Design review of the part shown in the three views and the two pictorial views. Dimensions are in mm from the part's minimum x, y and z. A direction names the side the tool comes from. Coordinates: 2 decimals unless noted, no trailing zeros. Loops run counter-clockwise (first coordinate to the right, second up) from the corner with the lowest first, then second, coordinate; pieces in that order, holes last. Notation, with made-up numbers: (68, 31) -> (79, 31) arc R23 ccw to (79, 69) -> close; hole circle Ø2 at (0, 46.5). An arc over 180 degrees is marked (long way). One line per item, written item: value.
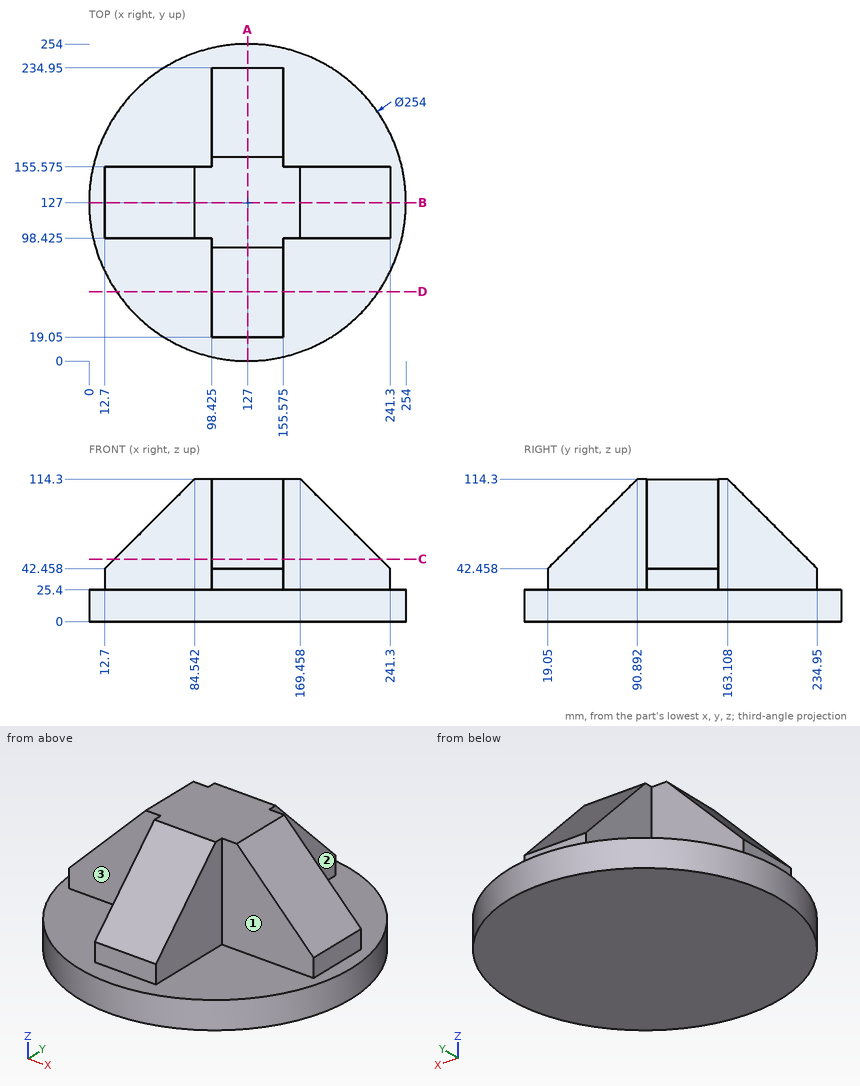
1. Take a section at C-C, the plane z = 50. Give the boundary of the cut face in (x, y) (3 decimals).
Return value:
outline: (20.242, 98.425) -> (98.425, 98.425) -> (98.425, 26.592) -> (155.575, 26.592) -> (155.575, 98.425) -> (233.758, 98.425) -> (233.758, 155.575) -> (155.575, 155.575) -> (155.575, 227.408) -> (98.425, 227.408) -> (98.425, 155.575) -> (20.242, 155.575) -> close
2. Take a section at D-D, the plane y = 55.5. Give the boundary of the cut face in (x, z) (3 decimals).
Return value:
outline: (22.039, 0) -> (231.961, 0) -> (231.961, 25.4) -> (155.575, 25.4) -> (155.575, 78.908) -> (98.425, 78.908) -> (98.425, 25.4) -> (22.039, 25.4) -> close
3. Insertion check: pin 1 Ø19 at (y, z) = (137, 30.5) entering from -X; pin 2 Ø19 at (x, z) = (123.5, 35) entering from -Y; pin 3 Ø2 at (y, z) = (185.5, 74.5) entering from +X (3 decimals). Each pin has a flat end and moves straight along its axis. Give the tip position at first contact, or say it passes through.
Return value:
pin 1: stops at x = 0.02
pin 2: stops at y = 19.05
pin 3: stops at x = 155.575
4. To check wall thickness, follow probe 1 along X at (y, z) = (72.5, 39.5) (3 decimals); probe 2 along Z at (x, y) = (211.5, 80). State the ranges of each line that lie inside material, in increasing order. Write a range as from..to.
Return value:
probe 1: x = 98.425..155.575
probe 2: z = 0..25.4
5. For the marked faces 1, 2 and 3, list the 3-axis set-ups (+Z, -Z, +X, -X, +Y, -Y) from which the entire face can be reached by the end or side of a thin tool; tool diameter is ignored.
Return value:
face 1: +Z, +X, -Y
face 2: +Z, +X, +Y
face 3: +Z, -X, -Y
6. Take a section at B-B, the plane y = 127. Give the boundary of the cut face in (x, z), and give its area (3 significant figures).
Return value:
outline: (0, 0) -> (254, 0) -> (254, 25.4) -> (241.3, 25.4) -> (241.3, 42.46) -> (169.46, 114.3) -> (84.54, 114.3) -> (12.7, 42.46) -> (12.7, 25.4) -> (0, 25.4) -> close
area: 21,600 mm2
7. Take a section at A-A, the plane x = 127. Give the boundary of the cut face in (y, z), and give its area (3 significant figures).
Return value:
outline: (0, 0) -> (254, 0) -> (254, 25.4) -> (234.95, 25.4) -> (234.95, 42.46) -> (163.11, 114.3) -> (90.89, 114.3) -> (19.05, 42.46) -> (19.05, 25.4) -> (0, 25.4) -> close
area: 20,500 mm2
